from build123d import *

# Parameters (mm, degrees)
SKIZZE1_R                       = 3.5
AUFSATZ_LINEAR_AUSTRAGEN1_DEPTH = 4
SKIZZE2_R                       = 1.95
AUFSATZ_LINEAR_AUSTRAGEN2_DEPTH = 12
FASE1_SIZE                      = 0.3
SCHNITT_LINEAR_AUSTRAGEN1_DEPTH = 2.5


with BuildPart() as part:
    # Skizze1 → Aufsatz-Linear austragen1 (new body)
    with BuildSketch(Plane.XY):
        Circle(SKIZZE1_R)
    extrude(amount=AUFSATZ_LINEAR_AUSTRAGEN1_DEPTH)

    # Skizze2 → Aufsatz-Linear austragen2 (add)
    with BuildSketch(Plane.XY.offset(4)):
        Circle(SKIZZE2_R)
    extrude(amount=AUFSATZ_LINEAR_AUSTRAGEN2_DEPTH)

    # Fase1
    fase1_edges = [part.edges().sort_by_distance(p)[0] for p in [
        (-3.5, 0, 0),
        (-3.5, 0, 4),
        (-1.95, 0, 16),
    ]]
    chamfer(fase1_edges, length=FASE1_SIZE)

    # Skizze3 → Schnitt-Linear austragen1 (cut)
    with BuildSketch(Plane(origin=(0, 0, 0), x_dir=(-1, 0, 0), z_dir=(0, 0, -1))):
        Polygon((1.5, 0.866025404), (0, 1.732050808), (-1.5, 0.866025404), (-1.5, -0.866025404), (0, -1.732050808), (1.5, -0.866025404), align=None)
    extrude(amount=-SCHNITT_LINEAR_AUSTRAGEN1_DEPTH, mode=Mode.SUBTRACT)


solid = part.part
Build history of the part. All positions in model axes, mm. A direction names the side the tool comes from. Coordinates: 2 decimals unless noted, no trailing zeros. Write each loop counter-clockwise with the first axis right and the second up, starting at its lowest first coordinate (ties: lowest second). Pieces come first, ordered by that corner, then holes.
(1) Drill centre lines: line 1 (Z direction, x = 2, y = 1.5); line 2 (Z direction, x = 0, y = 1.5); line 3 (X direction, y = -1.25, z = 2.25). Where is each one in solid material? Low to high.
(2) Cut at A-A on y = 0. List the corners of the cut face in (x, z).
(3) Mould opens along X. For faces 4 (the cylindrical face through (3.233, -1.341, 1.976)), 5 (the flat face through (0.76, -1.293, 1.232)), 6 (the flat face through (0, -2.1, 4)) say: pulls with the +X half, pulls with the -X half, needs draft (parallel to the pull), parting line crosses it, or undercut.
(4) Cut at B-B on z = 7.25. List the corners of the cut face in (x, y).
(5) 3-axis set-ups, long thin cutter, end or side, ignore diameter. For faces 1 (the flat face through (1.5, 0, 1)), 2 (the flat face through (-0.8, 1.5, 0)), 3 (the cylindrical face through (-1.437, 1.318, 9.768)): which of +Z, -Z, +X, -X, +Y, -Y reach the whole face in a straight line?
(6) Pin check, flat tip, straight feed: pin 1 Ø1.5 at (y, z) = (1.5, 14) entering from +X. Stop position of the tip, or through.
Working result:
1. line 1: z = 0 to 4
1. line 2: z = 2.5 to 16
1. line 3: x = -3.27 to -0.83, 0.83 to 3.27
2. outline: (-3.5, 0.3) - (-3.2, 0) - (-1.5, 0) - (-1.5, 2.5) - (1.5, 2.5) - (1.5, 0) - (3.2, 0) - (3.5, 0.3) - (3.5, 3.7) - (3.2, 4) - (1.95, 4) - (1.95, 15.7) - (1.65, 16) - (-1.65, 16) - (-1.95, 15.7) - (-1.95, 4) - (-3.2, 4) - (-3.5, 3.7) - close
3. face 4: parting line crosses it
3. face 5: undercut
3. face 6: needs draft
4. outline: circle Ø3.9 at (0, 0)
5. face 1: -Z
5. face 2: -Z, +X, -X, +Y, -Y
5. face 3: +Z
6. pin 1: stops at x = 1.8
